Design review of the part built by this model. Coordinates are the model's own, in mm. A direction names the side the tool comes from. Coordinates: 2 decimals unless noted, no trailing zeros. Write each loop counter-clockwise with the first axis right and the second up, starting at its lowest first coordinate (ties: lowest second). Pieces come first, ordered by that corner, then holes.
Q1. Clearance check with flat-ended pins moving along their axes: pin 1 Ø0.8 at (x, z) = (0.5, -19.5) entering from -Y; pin 2 Ø2.5 at (y, z) = (-6, 17.5) entering from -X; pin 3 Ø4 at (x, y) = (8, 17) entering from -Z; pin 4 Ø3 at (x, z) = (17, 17.5) entering from -Y. State where each tip first meets the part, or that it passes through.
Q2. Add section A-A, the plane x = 8.25. Give the boundary of the cut face in (y, z).
Q3. The part is to be moulded in two halves that separate along Z. For faces 1 (the face through (12.325, 20.861, -20.745)), 2 (the face through (2.07, -9.8, -13.76)), 3 (the face through (13, 16, 6)), say which applies: +Z half, -Z half, draft (parallel to the pull), parting line (faces both ways), or undercut.
Q4. Add section D-D, the plane y = 19. Give the boundary of the cut face in (x, z), plus the area to 3 significant figures.
Q5. Add section C-C, the plane z = 18. Give the boundary of the cut face in (x, y), plus the area to 3 significant figures.
Q6. Machinability: for faces 4 (the face through (2.05, -0.18, 16.93)), 5 (the face through (12.32, -14.45, -14.36)), which of the approach directions +Z, -Z, +X, -X, +Y, -Y give a long, thin tool a straight path to every point of the face, cutting with its end or side? Answer none if there is none.
Q7. Add section B-B, the plane y = -7. Give the boundary of the cut face in (x, z), plus the area to 3 significant figures.
Q8. To check wall thickness, follow probe 1 along Y at (x, z) = (6.25, 15.5); probe 2 along Z at (x, y) = (12.25, 0); probe 3 along Z at (x, y) = (21.25, 15). State the ranges of each line that lie inside material, in increasing order.
from build123d import *

# Parameters (mm, degrees)
CROQUIS1_R              = 11.1
CROQUIS1_R_2            = 1.55
SALIENTE_EXTRUIR1_DEPTH = 25
CORTAR_EXTRUIR1_DEPTH   = 42.024382994
CORTAR_EXTRUIR2_DEPTH   = 58.183913822


with BuildPart() as part:
    # Croquis1 → Saliente-Extruir1 (new body)
    with BuildSketch(Plane(origin=(0, 0, 0), x_dir=(0, 0, -1), z_dir=(1, 0, 0))):
        with BuildLine():
            Line((-15.5, 23), (15.5, 23))
            ThreePointArc((15.5, 23), (20.803300859, 20.803300859), (23, 15.5))
            Line((23, 15.5), (23, -15.5))
            ThreePointArc((23, -15.5), (20.803300859, -20.803300859), (15.5, -23))
            Line((15.5, -23), (-15.5, -23))
            ThreePointArc((-15.5, -23), (-20.803300859, -20.803300859), (-23, -15.5))
            Line((-23, -15.5), (-23, 15.5))
            ThreePointArc((-23, 15.5), (-20.803300859, 20.803300859), (-15.5, 23))
        make_face()
        Circle(CROQUIS1_R, mode=Mode.SUBTRACT)
        with Locations((-15.5, 15.5)):
            Circle(CROQUIS1_R_2, mode=Mode.SUBTRACT)
        with Locations((15.5, 15.5)):
            Circle(CROQUIS1_R_2, mode=Mode.SUBTRACT)
        with Locations((15.5, -15.5)):
            Circle(CROQUIS1_R_2, mode=Mode.SUBTRACT)
        with Locations((-15.5, -15.5)):
            Circle(CROQUIS1_R_2, mode=Mode.SUBTRACT)
    extrude(amount=SALIENTE_EXTRUIR1_DEPTH)

    # Croquis2 → Cortar-Extruir1 (cut, through all)
    with BuildSketch(Plane(origin=(25, 0, 0), x_dir=(0, 0, -1), z_dir=(1, 0, 0))):
        with BuildLine():
            Line((-6, 23), (-6, 9.33862945))
            ThreePointArc((-6, 9.33862945), (0, 11.1), (6, 9.33862945))
            Line((6, 9.33862945), (6, 23))
            Line((6, 23), (-6, 23))
        make_face()
    extrude(amount=-CORTAR_EXTRUIR1_DEPTH, mode=Mode.SUBTRACT)

    # Croquis3 → Cortar-Extruir2 (cut, through all)
    with BuildSketch(Plane(origin=(0, 0, -23), x_dir=(-1, 0, 0), z_dir=(0, 0, -1))):
        with BuildLine():
            Line((0, 0.25), (-1, 0.25))
            ThreePointArc((-1, 0.25), (-2.060660172, -0.189339828), (-2.5, -1.25))
            Line((-2.5, -1.25), (-2.5, -8.75))
            ThreePointArc((-2.5, -8.75), (-2.060660172, -9.810660172), (-1, -10.25))
            Line((-1, -10.25), (0, -10.25))
            Line((0, -10.25), (0, 0.25))
        make_face()
    extrude(amount=-CORTAR_EXTRUIR2_DEPTH, mode=Mode.SUBTRACT)


solid = part.part
Here are the results:
1. pin 1: stops at y = -22.08
1. pin 2: stops at x = 2.5
1. pin 3: stops at z = -23
1. pin 4: stops at y = -22.98
2. outline: (-23, -15.5) arc R7.5 ccw to (-15.5, -23) - (15.5, -23) arc R7.5 ccw to (23, -15.5) - (23, -6) - (9.34, -6) arc R11.1 cw (long way) to (9.34, 6) - (23, 6) - (23, 15.5) arc R7.5 ccw to (15.5, 23) - (-15.5, 23) arc R7.5 ccw to (-23, 15.5) - close; hole circle Ø3.1 at (-15.5, -15.5); hole circle Ø3.1 at (-15.5, 15.5); hole circle Ø3.1 at (15.5, -15.5); hole circle Ø3.1 at (15.5, 15.5)
3. face 1: -Z half
3. face 2: draft
3. face 3: undercut
4. outline: (0, -22.13) - (25, -22.13) - (25, -6) - (0, -6) - close; (0, 6) - (25, 6) - (25, 22.13) - (0, 22.13) - close
4. area: 807 mm2
5. outline: (0, -22.57) - (25, -22.57) - (25, 22.57) - (0, 22.57) - (0, 0.25) - (1, 0.25) arc R1.5 cw to (2.5, -1.25) - (2.5, -8.75) arc R1.5 cw to (1, -10.25) - (0, -10.25) - close
5. area: 1,100 mm2
6. face 4: +Z, -Z, -X
6. face 5: +X, -X
7. outline: (2.5, -23) - (25, -23) - (25, -8.61) - (2.5, -8.61) - close; (2.5, 8.61) - (25, 8.61) - (25, 23) - (2.5, 23) - close
7. area: 647 mm2
8. probe 1: y = -23 to -17.05, -13.95 to 13.95, 17.05 to 23
8. probe 2: z = -23 to -11.1, 11.1 to 23
8. probe 3: z = -23 to -16.97, -14.03 to -6, 6 to 14.03, 16.97 to 23
